Part model, mm, in its own coordinate system. A direction names the side the tool comes from. Coordinates: 2 decimals unless noted, no trailing zeros. Loops run counter-clockwise (first coordinate to the right, second up) from the corner with the lowest first, then second, coordinate; pieces in that order, holes last. Notation, with made-up numbers: (-4.75, 57) - (39.25, 57) arc R17 cw to (39.25, 89) - close; hole circle Ø10 at (87.5, 44.25). An arc over 180 degrees is marked (long way). Use a Markdown table: item, result. Add a question column.
1. Band-saw the part on B-B, the plane y = 131.5. Give the cut face in (x, z), plus the area to 3 significant figures.
2. 3-axis set-ups, long thin cutter, end or side, ignore diameter. For faces 1 (the flat face through (491, -460, -17)), 2 (the flat face through (-6, 460, -23)), 3 (the flat face through (-490, -6, -23)), 4 (the flat face through (-6, -83, 3)): which of +Z, -Z, +X, -X, +Y, -Y reach the whole face in a straight line?
3. Band-saw the part on C-C, the plane x = 368.5. Give the cut face in (y, z), plus the area to 3 significant figures.
4. Band-saw the part on A-A, the plane z = 76.5. Give the cut face in (x, y).
5. Pull direction X, two halves, no side cores. Call faces 5 (the flat face through (-500, -6, -22)), 6 (the flat face through (312, 253, 95)), 7 (the cylindrical face through (-14.985, -0.66, -24.65)): pulls with the +X half, pulls with the -X half, needs draft (parallel to the pull), parting line crosses it, or undercut.
6. Drop flat-ended pins along their axis: pin 1 (3 mm diameter, centred on y = 467, z = -33, fed in from -X); pin 2 (2 mm diameter, centred on x = 175, z = 60.5, fed in from -Y); pin 3 (1 mm diameter, centred on x = 71.5, z = 4.5, fed in from +Y). Give the stop position or say it passes through.
7. Wall check: probe 1 along Y at (x, z) = (-470, 1); probe 2 along X at (y, z) = (-319.5, -42.5); probe 3 along Y at (x, z) = (-143, -20.5). Give the ranges that are in metal, low to high. Write a range as [from, to].
from build123d import *

# Parameters (mm, degrees)
F2_W     = 1000
F2_H     = 920
F2_R     = 10
F2_R_2   = 401
F3_DEPTH = 3
F4_W     = 890
F4_H     = 10
F4_W_2   = 10
F4_H_2   = 920
F5_DEPTH = 50
F6_R     = 15
F6_R_2   = 10
F7_DEPTH = 50


with BuildPart() as f1:
    # F0 (on Front) → F1 (revolve)
    with BuildSketch(Plane.XZ):
        Polygon((-425, 3), (-400, 3), (-400, 55), (-401, 55), (-401, 95), (-424, 95), (-424, 55), (-425, 55), align=None)
        Polygon((-10, 3), (-400, 3), (-425, 3), (-425, 0), (-10, 0), align=None)
    revolve(axis=Axis((0, 0, 187.921241), (0, 0, -1)))

    # F2 (on Top) → F3 (join)
    with BuildSketch(Plane.XY):
        Rectangle(F2_W, F2_H)
        with Locations((-470, -430)):
            Circle(F2_R, mode=Mode.SUBTRACT)
        with Locations((470, -430)):
            Circle(F2_R, mode=Mode.SUBTRACT)
        with Locations((-470, 430)):
            Circle(F2_R, mode=Mode.SUBTRACT)
        Circle(F2_R_2, mode=Mode.SUBTRACT)
        with Locations((470, 430)):
            Circle(F2_R, mode=Mode.SUBTRACT)
    extrude(amount=F3_DEPTH)

    # F4 (on face) → F5 (join)
    with BuildSketch(Plane.XY.offset(3)):
        with Locations((0, -465)):
            Rectangle(F4_W, F4_H)
        with Locations((-495, 0)):
            Rectangle(F4_W_2, F4_H_2)
        with Locations((0, 465)):
            Rectangle(F4_W, F4_H)
        with Locations((495, 0)):
            Rectangle(F4_W_2, F4_H_2)
    extrude(amount=-F5_DEPTH)

    # F6 (on face) → F7 (join)
    with BuildSketch(Plane(origin=(0, 0, 0), x_dir=(1, 0, 0), z_dir=(0, 0, -1))):
        Circle(F6_R)
        Circle(F6_R_2, mode=Mode.SUBTRACT)
    extrude(amount=F7_DEPTH)


solid = f1.part
Geometry check:
| question | item | result |
|---|---|---|
| 1 | outline | (-500, -47) - (-490, -47) - (-490, 0) - (490, 0) - (490, -47) - (500, -47) - (500, 3) - (404.14, 3) - (404.14, 55) - (403.09, 55) - (403.09, 95) - (378.83, 95) - (378.83, 55) - (377.77, 55) - (377.77, 3) - (-377.77, 3) - (-377.77, 55) - (-378.83, 55) - (-378.83, 95) - (-403.09, 95) - (-403.09, 55) - (-404.14, 55) - (-404.14, 3) - (-500, 3) - close |
| 1 | area | 8,620 mm^2 |
| 2 | face 1 | +Z, -Z, +X, -Y |
| 2 | face 2 | -Z |
| 2 | face 3 | -Z, +Y, -Y |
| 2 | face 4 | +Z |
| 3 | outline | (-470, -47) - (-460, -47) - (-460, 0) - (460, 0) - (460, -47) - (470, -47) - (470, 3) - (211.74, 3) - (211.74, 55) - (209.72, 55) - (209.72, 95) - (158.14, 95) - (158.14, 55) - (155.59, 55) - (155.59, 3) - (-155.59, 3) - (-155.59, 55) - (-158.14, 55) - (-158.14, 95) - (-209.72, 95) - (-209.72, 55) - (-211.74, 55) - (-211.74, 3) - (-470, 3) - close |
| 3 | area | 13,700 mm^2 |
| 4 | outline | circle Ø848 at (0, 0); hole circle Ø802 at (0, 0) |
| 5 | face 5 | pulls with the -X half |
| 5 | face 6 | needs draft |
| 5 | face 7 | undercut |
| 6 | pin 1 | stops at x = -445 |
| 6 | pin 2 | stops at y = -386.65 |
| 6 | pin 3 | stops at y = 419.03 |
| 7 | probe 1 | y = [-460, -440], [-420, 420], [440, 460] |
| 7 | probe 2 | x = [-500, -490], [490, 500] |
| 7 | probe 3 | y = [-470, -460], [460, 470] |
